Input: part model. Units: mm. Frame: model coordinates. Coordinates: 2 decimals unless noted, no trailing zeros. Loops run counter-clockwise (first coordinate to the right, second up) from the corner with the lowest first, then second, coordinate; pieces in that order, holes last. Notation, with made-up numbers: M 34,54.25 L 53,54.25 A14 cw 53,65.25 Z; hole C 43.25,-32.75 d8. An arc over 180 degrees is marked long. Use a Markdown table: item, result. Add a question column.
1. Section B-B on y = 19. Output: boundary loops of the cut face in (x, z).
2. Section C-C on z = 1.5. State how many separate pieces and enclosed holes the cut face has, then the cut area to 3 significant figures.
3. Line query: L1, parallel to X at y = 71.5, z = 0.85; L2, parallel to X at y = -82, z = 1.5; L3, parallel to Y at x = -20, z = 2. Output: solid intervals per line, ascending. Write a range as [from, to].
4. Section A-A on x = -9.5. Output: boundary loops of the cut face in (y, z).
5. Pin query (flat end, axial travel): pin 1 (3 mm diameter, centred on x = 102, y = -82, fed in from +Z). Return the tip coordinate at first contact, or that it passes through.
Solid Edge part; units mm, degrees
sketch "Sketch1" plane through (0, 0, 0) normal (0, 0, 1) x (1, 0, 0)
  line L0 (-110, -90) -> (110, -90)
  line L1 (110, -90) -> (110, 90)
  line L2 (110, 90) -> (-110, 90)
  line L3 (-110, 90) -> (-110, -90)
  circle A0 centre (-20, 0) radius 32.3
  circle A1 centre (-102, -82) radius 1.7
  circle A2 centre (-102, 82) radius 1.7
  circle A3 centre (102, -82) radius 1.7
  circle A4 centre (102, 82) radius 1.7
  circle A5 centre (0, -82) radius 1.7
  circle A6 centre (0, 82) radius 1.7
  circle A7 centre (17, 0) radius 1.7
  circle A8 centre (-57, 0) radius 1.7
  circle A9 centre (-20, 37) radius 1.7
  circle A10 centre (-20, -37) radius 1.7
  circle A11 centre (51.3137, 11.3137) radius 1.7
  circle A12 centre (28.6863, 11.3137) radius 1.7
  circle A13 centre (28.6863, -11.3137) radius 1.7
  circle A14 centre (51.3137, -11.3137) radius 1.7
  line L4 (-80, 58) -> (-75, 58)
  line L5 (-75, 58) -> (-75, 78)
  line L6 (-75, 78) -> (-80, 78)
  line L7 (-80, 78) -> (-80, 58)
  line L8 (-68, 58) -> (-63, 58)
  line L9 (-63, 58) -> (-63, 78)
  line L10 (-63, 78) -> (-68, 78)
  line L11 (-68, 78) -> (-68, 58)
  line L12 (-56, 58) -> (-51, 58)
  line L13 (-51, 58) -> (-51, 78)
  line L14 (-51, 78) -> (-56, 78)
  line L15 (-56, 78) -> (-56, 58)
  line L16 (-44, 58) -> (-39, 58)
  line L17 (-39, 58) -> (-39, 78)
  line L18 (-39, 78) -> (-44, 78)
  line L19 (-44, 78) -> (-44, 58)
  line L20 (-32, 58) -> (-27, 58)
  line L21 (-27, 58) -> (-27, 78)
  line L22 (-27, 78) -> (-32, 78)
  line L23 (-32, 78) -> (-32, 58)
extrude "Protrusion1" add sketch "Sketch1" along normal blind 5
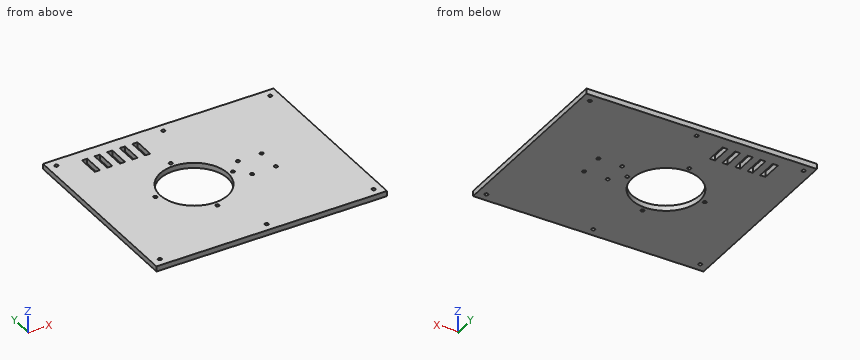
Answers below:
| question | item | result |
|---|---|---|
| 1 | outline | M -110,0 L -46.12,0 L -46.12,5 L -110,5 Z; M 6.12,0 L 110,0 L 110,5 L 6.12,5 Z |
| 2 | separate pieces | 1 |
| 2 | enclosed holes | 20 |
| 2 | area | 35,700 mm² |
| 3 | L1 | x = [-110, -80], [-75, -68], [-63, -56], [-51, -44], [-39, -32], [-27, 110] |
| 3 | L2 | x = [-110, -103.7], [-100.3, -1.7], [1.7, 100.3], [103.7, 110] |
| 3 | L3 | y = [-90, -38.7], [-35.3, -32.3], [32.3, 35.3], [38.7, 90] |
| 4 | outline | M -90,0 L -30.55,0 L -30.55,5 L -90,5 Z; M 30.55,0 L 90,0 L 90,5 L 30.55,5 Z |
| 5 | pin 1 | passes through |
